```python
from build123d import *

# Parameters (mm, degrees)
SKETCH1_W            = 180
SKETCH1_H            = 120
BOSS_EXTRUDE1_DEPTH  = 20
SKETCH4_W            = 180
SKETCH4_H            = 100
BOSS_EXTRUDE4_DEPTH  = 20
BOSS_EXTRUDE5_DEPTH  = 20
SKETCH6_R            = 6.4
BOSS_EXTRUDE11_DEPTH = 80


with BuildPart() as part:
    # Sketch1 → Boss-Extrude1 (new body)
    with BuildSketch(Plane.XY):
        Rectangle(SKETCH1_W, SKETCH1_H)
    extrude(amount=BOSS_EXTRUDE1_DEPTH)

    # Sketch4 → Boss-Extrude4 (add)
    with BuildSketch(Plane(origin=(0, -60, 0), x_dir=(-1, 0, 0), z_dir=(0, -1, 0))):
        with Locations((0, -50)):
            Rectangle(SKETCH4_W, SKETCH4_H)
    extrude(amount=-BOSS_EXTRUDE4_DEPTH)

    # Sketch5 → Boss-Extrude5 (add)
    with BuildSketch(Plane(origin=(90, 0, 0), x_dir=(0, 0, -1), z_dir=(1, 0, 0))):
        Polygon((-100, -40), (-20, -40), (-20, 60), align=None)
    boss_extrude5 = extrude(amount=-BOSS_EXTRUDE5_DEPTH)

    # Mirror2: Boss-Extrude5 across plane
    add(boss_extrude5.mirror(Plane(origin=(0, 0, 0), x_dir=(0, 0, 1), z_dir=(1, 0, 0))))

    # Sketch6 → Boss-Extrude11 (add)
    with BuildSketch(Plane.XY.offset(20)):
        with BuildLine():
            Line((-41.754337398, -40), (-58.837662602, -40))
            ThreePointArc((-58.837662602, -40), (-50.296, -9.6), (-41.754337398, -40))
        make_face()
        with Locations((-50.296, -26)):
            Circle(SKETCH6_R, mode=Mode.SUBTRACT)
    boss_extrude11 = extrude(amount=BOSS_EXTRUDE11_DEPTH)

    # Mirror3: Boss-Extrude11 across plane
    add(boss_extrude11.mirror(Plane(origin=(0, 0, 0), x_dir=(0, 0, 1), z_dir=(1, 0, 0))))


solid = part.part
```
Design review of the part built by this model. Coordinates are the model's own, in mm. A direction names the side the tool comes from. Coordinates: 2 decimals unless noted, no trailing zeros. Order: outer loops, then holes, each group sorted by start corner. A loop starts at its lowest first (then second) coordinate and runs counter-clockwise, first axis right, second up.
1) Clearance check with flat-ended pins moving along their axes: pin 1 (12.5 mm diameter, centred on x = -63.5, z = 49.5, fed in from +Y); pin 2 (24 mm diameter, centred on x = -1.5, z = 59, fed in from +Y); pin 3 (2 mm diameter, centred on x = -6.5, y = 15, fed in from +Z). State where each tip first meets the part, or that it passes through.
2) Take a section at B-B, the plane y = 34. Give the boundary of the cut face in (x, z).
3) Take a section at D-D, the plane z = 67. Give the boundary of the cut face in (x, y).
4) Mouldability with a two-part tool opening along X and no side actions: class faces 1 (the flat face through (-90, -12, 40)), 2 (the cylindrical face through (-50.89, -9.61, 59.44)), 3 (the flat face through (-1, 1, 0)) as +X half, -X half, draft (parallel to the pull), parting line (faces both ways), or undercut.
5) Take a section at C-C, the plane x = 5.5. Give the boundary of the cut face in (y, z).
6) Wall thickness on line 1 along X through (y, z) = (15, 43); line 2 along X through (y, z) = (-13, 71.5); line 3 along Y through (x, z) = (-36.5, 57.5): over which ranges is each line inside the solid? List them lowest first.
7) Take a section at A-A, the plane z = 24. Give the boundary of the cut face in (x, y), and give its area (3 significant figures).
8) For faces 4 (the flat face through (70, -12, 43)), 5 (the flat face through (-80.14, 10.7, 59.44)), 6 (the flat face through (1, -40, 59)), list the 3-axis set-ups (+Z, -Z, +X, -X, +Y, -Y) from which the entire face can be reached by the end or side of a thin tool; tool diameter is ignored.
Returned:
1. pin 1: stops at y = -11.15
1. pin 2: stops at y = -40
1. pin 3: stops at z = 20
2. outline: (-90, 0) - (90, 0) - (90, 40.8) - (70, 40.8) - (70, 20) - (-70, 20) - (-70, 40.8) - (-90, 40.8) - close
3. outline: (-90, -60) - (90, -60) - (90, 1.25) - (70, 1.25) - (70, -40) - (58.84, -40) arc R16.4 ccw (long way) to (41.75, -40) - (-41.75, -40) arc R16.4 ccw (long way) to (-58.84, -40) - (-70, -40) - (-70, 1.25) - (-90, 1.25) - close; hole circle Ø12.8 at (-50.3, -26); hole circle Ø12.8 at (50.3, -26)
4. face 1: -X half
4. face 2: undercut
4. face 3: draft
5. outline: (-60, 0) - (60, 0) - (60, 20) - (-40, 20) - (-40, 100) - (-60, 100) - close
6. line 1: x = -90 to -70, 70 to 90
6. line 2: x = -90 to -70, -60.29 to -40.3, 40.3 to 60.29, 70 to 90
6. line 3: y = -60 to -40, -34.87 to -17.13
7. outline: (-90, -60) - (90, -60) - (90, 55) - (70, 55) - (70, -40) - (58.84, -40) arc R16.4 ccw (long way) to (41.75, -40) - (-41.75, -40) arc R16.4 ccw (long way) to (-58.84, -40) - (-70, -40) - (-70, 55) - (-90, 55) - close; hole circle Ø12.8 at (-50.3, -26); hole circle Ø12.8 at (50.3, -26)
7. area: 8,780 mm2
8. face 4: +Z, +Y
8. face 5: +Z, -X, +Y
8. face 6: +Z
